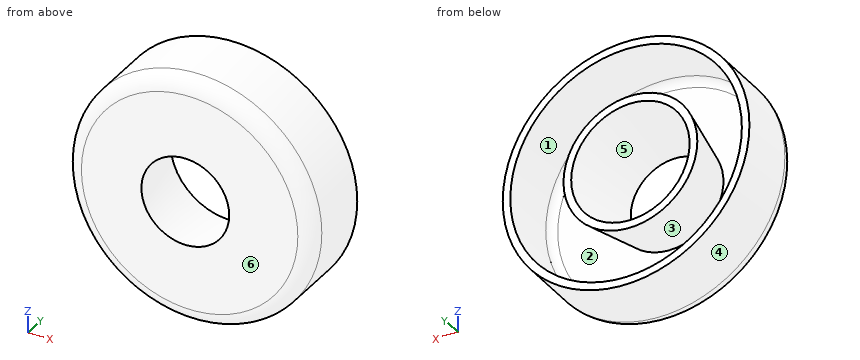
```python
from build123d import *

# Parameters (mm, degrees)
F1_R     = 40.7423360253
F2_DEPTH = 25
F3_R     = 19.5601176406
F4_R     = 14.5028723408
F6_R     = 5
F7_T     = -2.5


with BuildPart() as f2:
    # F1 (on Front) → F2 (new body)
    with BuildSketch(Plane.XZ):
        with Locations((1.4253406553, 0)):
            Circle(F1_R)
    extrude(amount=F2_DEPTH)

    # F3 (on Front) → F5 section 0
    with BuildSketch(Plane.XZ):
        Circle(F3_R)
    # F4 (on offset) → F5 section 1
    with BuildSketch(Plane.XZ.offset(25)):
        Circle(F4_R)
    loft(mode=Mode.SUBTRACT)

    # F6
    f6_edges = [f2.edges().sort_by_distance(p)[0] for p in [
        (-39.316995, -25, 0),
    ]]
    fillet(f6_edges, radius=F6_R)

    # F7
    f7_openings = [f2.faces().sort_by_distance(p)[0] for p in [
        (-38.164628, 0, 0),
    ]]
    offset(amount=F7_T, openings=f7_openings, kind=Kind.INTERSECTION)


solid = f2.part
```
CAD build for the part. Positions are in the model's coordinates, mm. Face numbers are marked on the shaded views. A direction names the side the tool comes from. Coordinates: 2 decimals unless noted, no trailing zeros. Loops run counter-clockwise (first coordinate to the right, second up) from the corner with the lowest first, then second, coordinate; pieces in that order, holes last. Notation, with made-up numbers: (-1.5, 84) - (10.5, 84) arc R10 cw to (10.5, 93) - close; hole circle Ø7 at (-29.5, -21). An arc over 180 degrees is marked (long way). Return JSON: item names as keys, results as strings.
1. Drop flat-ended pins along their axis: pin 1 (4 mm diameter, centred on x = 22, z = 20, fed in from +Y); pin 2 (10 mm diameter, centred on y = -20, z = -6, fed in from -X); pin 3 (6 mm diameter, centred on y = -9.5, z = 26.5, fed in from -X). Give the stop position or say it passes through.
Result:
{"pin 1": "stops at y = -22.5", "pin 2": "stops at x = -39.3", "pin 3": "stops at x = -31.86"}
2. Band-saw the part on A-A (y = -13.75). Give the cut face in (x, z).
Result:
{"outline": "circle Ø81.48 at (1.43, 0); circle Ø38.66 at (0, 0); hole circle Ø76.48 at (1.43, 0); hole circle Ø33.56 at (0, 0)"}
3. Probe L1, parallel to Z at x = -14, y = -14.25; L2, parallel to X at y = -18.75, z = 1; L3, parallel to X at y = -7, z = -18.5. List the from-to ranges inside material, lowest first. Write a range as from..to.
Result:
{"L1": "z = -37.71..-34.99, -13.18..-9.06, 9.06..13.18, 34.99..37.71", "L2": "x = -39.3..-36.8, -18.29..-15.74, 15.74..18.29, 39.65..42.16", "L3": "x = -34.87..-32.04, -9.27..9.27, 34.9..37.73"}
4. Mould opens along Y. For the marked faces 3, 4, 5 and 6 say: released by +Y, released by -Y, zero draft, split by the parting line, or undercut.
Result:
{"face 3": "undercut", "face 4": "zero draft", "face 5": "released by +Y", "face 6": "released by -Y"}
5. Band-saw the part on B-B (y = -1.75). Give the cut face in (x, z).
Result:
{"outline": "circle Ø81.48 at (1.43, 0); circle Ø43.51 at (0, 0); hole circle Ø76.48 at (1.43, 0); hole circle Ø38.41 at (0, 0)"}
6. 3-axis set-ups, long thin cutter, end or side, ignore diameter. For the marked faces 1 and 2: which of +Z, -Z, +X, -X, +Y, -Y reach the whole face in a straight line?
Result:
{"face 1": "+Y", "face 2": "none"}
